CAD build for the part. Positions are in the model's coordinates, mm. A direction names the side the tool comes from. Coordinates: 2 decimals unless noted, no trailing zeros. Order: outer loops, then holes, each group sorted by start corner. A loop starts at its lowest first (then second) coordinate and runs counter-clockwise, first axis right, second up. Notation, with made-up numbers: (79.25, -36.75) - (84.25, -36.75) arc R25 ccw to (84.25, -9.75) - close; hole circle Ø7 at (-16, 67.5). An arc over 180 degrees is marked (long way). Return JSON: item names as keys, results as strings.
from build123d import *

# Parameters (mm, degrees)
F1_DEPTH = 8


with BuildPart() as f1:
    # F0 (on Front) → F1 (new body, symmetric)
    with BuildSketch(Plane.XZ):
        with BuildLine():
            Line((-23.820377, -11.462722), (24.179623, -11.462722))
            Line((24.179623, -11.462722), (23.863268, -4.417862))
            ThreePointArc((23.863268, -4.417862), (23.555339, -3.739929), (22.864275, -3.462722))
            Line((22.864275, -3.462722), (13.5, -3.462722))
            ThreePointArc((13.5, -3.462722), (12.792893, -3.169829), (12.5, -2.462722))
            Line((12.5, -2.462722), (12.5, 31.537278))
            ThreePointArc((12.5, 31.537278), (12.207107, 32.244384), (11.5, 32.537278))
            Line((11.5, 32.537278), (1.5, 32.537278))
            Line((1.5, 32.537278), (1.5, 25.395395))
            ThreePointArc((1.5, 25.395395), (0, 9.537278), (-1.5, 25.395395))
            Line((-1.5, 25.395395), (-1.5, 32.537278))
            Line((-1.5, 32.537278), (-11.5, 32.537278))
            ThreePointArc((-11.5, 32.537278), (-12.207107, 32.244384), (-12.5, 31.537278))
            Line((-12.5, 31.537278), (-12.5, -2.462722))
            ThreePointArc((-12.5, -2.462722), (-12.792893, -3.169829), (-13.5, -3.462722))
            Line((-13.5, -3.462722), (-22.820377, -3.462722))
            ThreePointArc((-22.820377, -3.462722), (-23.527483, -3.755616), (-23.820377, -4.462722))
            Line((-23.820377, -4.462722), (-23.820377, -11.462722))
        make_face()
    extrude(amount=F1_DEPTH, both=True)


solid = f1.part
Item 1: Which spindle directions (+Z, -Z, +X, -X, +Y, -Y) get a long thin tool onto all of the face, cutting with end or side? Do faces 4 (the flat face through (-1.5, 0, 29)), 5 (the flat face through (12.5, 0, 14)), 6 (the flat face through (-12.5, 0, 15)). Say none if no direction does.
Findings below:
{"face 4": "+Z, +Y, -Y", "face 5": "+Z, +X, +Y, -Y", "face 6": "+Z, -X, +Y, -Y"}
Item 2: Band-saw the part on B-B, the plane x = -3. List the corners of the cut face in (y, z).
Findings below:
{"outline": "(-8, -11.46) - (8, -11.46) - (8, 10.12) - (-8, 10.12) - close; (-8, 24.95) - (8, 24.95) - (8, 32.54) - (-8, 32.54) - close"}
Item 3: Drop flat-ended pins along their axis: P1, Ø12, axis at x = -15, z = 2, coming from the -Y side; P2, Ø5, axis at y = -5, z = 8, coming from the -X side; P3, Ø2, axis at y = 3.5, z = 6, coming from the +X side; P4, Ø9.5, axis at x = 0, z = 17.54, coming from the -Y side. Give the stop position or say it passes through.
Findings below:
{"P1": "stops at y = -8", "P2": "stops at x = -12.5", "P3": "stops at x = 12.5", "P4": "passes through"}
Item 4: Band-saw the part on D-D, the plane x = -21. List the corners of the cut face in (y, z), then the cut area to 3 significant figures.
Findings below:
{"outline": "(-8, -11.46) - (8, -11.46) - (8, -3.46) - (-8, -3.46) - close", "area": "128 mm²"}
Item 5: Band-saw the part on C-C, the plane y = -7. List the corners of the cut face in (x, z).
Findings below:
{"outline": "(-23.82, -11.46) - (24.18, -11.46) - (23.86, -4.42) arc R1 ccw to (22.86, -3.46) - (13.5, -3.46) arc R1 cw to (12.5, -2.46) - (12.5, 31.54) arc R1 ccw to (11.5, 32.54) - (1.5, 32.54) - (1.5, 25.4) arc R8 cw (long way) to (-1.5, 25.4) - (-1.5, 32.54) - (-11.5, 32.54) arc R1 ccw to (-12.5, 31.54) - (-12.5, -2.46) arc R1 cw to (-13.5, -3.46) - (-22.82, -3.46) arc R1 ccw to (-23.82, -4.46) - close"}
Item 6: Band-saw the part on A-A, the plane z = 28.5. List the corners of the cut face in (x, y).
Findings below:
{"outline": "(-12.5, -8) - (-1.5, -8) - (-1.5, 8) - (-12.5, 8) - close; (1.5, -8) - (12.5, -8) - (12.5, 8) - (1.5, 8) - close"}
Item 7: Wall check: L1, parallel to Z at x = 17.5, y = 0.25; L2, parallel to X at y = 1.75, z = 6; L3, parallel to X at y = -4, z = 26.5. Give the ranges that are in metal, low to high. Write a range as [from, to].
Findings below:
{"L1": "z = [-11.46, -3.46]", "L2": "x = [-12.5, 12.5]", "L3": "x = [-12.5, -1.5], [1.5, 12.5]"}
Item 8: Mould opens along Z. For faces 1 (the flat face through (7, 0, 32.537)), 2 (the cylindrical face through (0.331, -0.112, 9.544)), 3 (the flat face through (0, 8, 6)) say: released by +Z, released by -Z, zero draft, split by the parting line, or undercut.
Findings below:
{"face 1": "released by +Z", "face 2": "undercut", "face 3": "zero draft"}
